from build123d import *

# Parameters (mm, degrees)
SKETCH2_R           = 3.0099
BOSS_EXTRUDE1_DEPTH = 6.0198
SKETCH3_R           = 4.5466
SKETCH3_W           = 6.223
SKETCH3_H           = 8.4836
BOSS_EXTRUDE2_DEPTH = 0.9398
SKETCH4_R           = 4.5466
BOSS_EXTRUDE3_DEPTH = 17.6022
SKETCH5_W           = 6.223
SKETCH5_H           = 8.4836
CUT_EXTRUDE1_DEPTH  = 1.8542
SKETCH6_R           = 5.969
BOSS_EXTRUDE4_DEPTH = 1.8542
SKETCH9_R           = 6.985
BOSS_EXTRUDE6_DEPTH = 2.5654
DRAFT2_ANGLE        = -25
DRAFT3_ANGLE        = -25
SKETCH12_R          = 3.8989
BOSS_EXTRUDE7_DEPTH = 25.654


with BuildPart() as part:
    # Sketch2 → Boss-Extrude1 (new body)
    with BuildSketch(Plane(origin=(0, 0, 0), x_dir=(0, 0, -1), z_dir=(1, 0, 0))):
        with BuildLine():
            ThreePointArc((-32.512356648, -30.822448246), (-32.069394739, -31.178374506), (-31.515555535, -31.3055))
            Line((-31.515555535, -31.3055), (-29.21, -31.3055))
            ThreePointArc((-29.21, -31.3055), (-28.311974388, -30.933525612), (-27.94, -30.0355))
            Line((-27.94, -30.0355), (-27.94, -23.3045))
            ThreePointArc((-27.94, -23.3045), (-24.700446352, -20.987224463), (-22.998148855, -17.3863))
            Line((-22.998148855, -17.3863), (-22.998148855, -11.1633))
            Line((-22.998148855, -11.1633), (-24.8285, -11.1633))
            Line((-24.8285, -11.1633), (-24.8285, -4.3815))
            Line((-24.8285, -4.3815), (-21.082, -4.3815))
            Line((-21.082, -4.3815), (-21.082, 11.6205))
            Line((-21.082, 11.6205), (-10.8966, 19.2405))
            Line((-10.8966, 19.2405), (10.8966, 19.2405))
            Line((10.8966, 19.2405), (21.082, 11.6205))
            Line((21.082, 11.6205), (21.082, -4.3815))
            Line((21.082, -4.3815), (24.8285, -4.3815))
            Line((24.8285, -4.3815), (24.8285, -11.1633))
            Line((24.8285, -11.1633), (22.998148855, -11.1633))
            Line((22.998148855, -11.1633), (22.998148855, -17.3863))
            ThreePointArc((22.998148855, -17.3863), (24.700446352, -20.987224463), (27.94, -23.3045))
            Line((27.94, -23.3045), (27.94, -30.0355))
            ThreePointArc((27.94, -30.0355), (28.311974388, -30.933525612), (29.21, -31.3055))
            Line((29.21, -31.3055), (31.515555535, -31.3055))
            ThreePointArc((31.515555535, -31.3055), (32.069394739, -31.178374506), (32.512356648, -30.822448246))
            Line((32.512356648, -30.822448246), (42.536992541, -18.124576114))
            ThreePointArc((42.536992541, -18.124576114), (43.315187388, -16.736717659), (43.625872471, -15.176200729))
            Line((43.625872471, -15.176200729), (44.800437362, 14.721814671))
            ThreePointArc((44.800437362, 14.721814671), (43.830873172, 17.911699115), (41.092535101, 19.813519845))
            Line((41.092535101, 19.813519845), (6.15681953, 29.583677589))
            ThreePointArc((6.15681953, 29.583677589), (0, 30.428383513), (-6.15681953, 29.583677589))
            Line((-6.15681953, 29.583677589), (-41.092535101, 19.813519845))
            ThreePointArc((-41.092535101, 19.813519845), (-43.830873172, 17.911699115), (-44.800437362, 14.721814671))
            Line((-44.800437362, 14.721814671), (-43.625872471, -15.176200729))
            ThreePointArc((-43.625872471, -15.176200729), (-43.315187388, -16.736717659), (-42.536992541, -18.124576114))
            Line((-42.536992541, -18.124576114), (-32.512356648, -30.822448246))
        make_face()
        with Locations((-34.798, 10.8585)):
            Circle(SKETCH2_R, mode=Mode.SUBTRACT)
        with Locations((34.798, 10.8585)):
            Circle(SKETCH2_R, mode=Mode.SUBTRACT)
    extrude(amount=BOSS_EXTRUDE1_DEPTH)

    # Sketch3 → Boss-Extrude2 (add)
    with BuildSketch(Plane(origin=(6.0198, 0, 0), x_dir=(0, 0, -1), z_dir=(1, 0, 0))):
        with Locations((33.9979, -16.616175495)):
            Circle(SKETCH3_R)
        with Locations((-33.9979, -16.616175495)):
            Circle(SKETCH3_R)
        with Locations((24.1935, 2.6543)):
            Rectangle(SKETCH3_W, SKETCH3_H)
        with Locations((-24.1935, 2.6543)):
            Rectangle(SKETCH3_W, SKETCH3_H)
    extrude(amount=BOSS_EXTRUDE2_DEPTH)

    # Sketch4 → Boss-Extrude3 (add)
    with BuildSketch(Plane(origin=(6.9596, 0, 0), x_dir=(0, 0, -1), z_dir=(1, 0, 0))):
        with Locations((-33.9979, -16.616175495)):
            Circle(SKETCH4_R)
        with Locations((33.9979, -16.616175495)):
            Circle(SKETCH4_R)
    extrude(amount=BOSS_EXTRUDE3_DEPTH)

    # Sketch5 → Cut-Extrude1 (cut)
    with BuildSketch(Plane.ZY):
        with Locations((-24.1935, 2.6543)):
            Rectangle(SKETCH5_W, SKETCH5_H)
        with Locations((24.1935, 2.6543)):
            Rectangle(SKETCH5_W, SKETCH5_H)
    extrude(amount=-CUT_EXTRUDE1_DEPTH, mode=Mode.SUBTRACT)

    # Sketch6 → Boss-Extrude4 (add)
    with BuildSketch(Plane.ZY):
        with Locations(Location((33.9979, -16.616175495, 0), (0, 0, 180))):
            Circle(SKETCH6_R)
        with Locations(Location((-33.9979, -16.616175495, 0), (0, 0, 180))):
            Circle(SKETCH6_R)
    extrude(amount=BOSS_EXTRUDE4_DEPTH)

    # Sketch9 → Boss-Extrude6 (add)
    with BuildSketch(Plane.ZY.offset(1.8542)):
        with Locations((33.9979, -16.616175495)):
            Circle(SKETCH9_R)
        with Locations(Location((-33.9979, -16.616175495, 0), (0, 0, 180))):
            Circle(SKETCH9_R)
    extrude(amount=BOSS_EXTRUDE6_DEPTH)

    # Draft2
    draft2_faces = [part.faces().sort_by_distance(p)[0] for p in [
        (-3.1369, -16.616175495, -27.0129),
    ]]
    draft(draft2_faces, Plane(origin=(-1.8542, -16.616175495, -33.9979), x_dir=(0, 0, 1), z_dir=(1, 0, 0)), DRAFT2_ANGLE)

    # Draft3
    draft3_faces = [part.faces().sort_by_distance(p)[0] for p in [
        (-3.1369, -16.616175495, 27.0129),
    ]]
    draft(draft3_faces, Plane(origin=(-1.8542, -16.616175495, 33.9979), x_dir=(0, 0, 1), z_dir=(1, 0, 0)), DRAFT3_ANGLE)

    # Sketch12 → Boss-Extrude7 (add)
    with BuildSketch(Plane.ZY.offset(4.4196)):
        with Locations((-33.9979, -16.616175495)):
            Circle(SKETCH12_R)
        with Locations(Location((33.9979, -16.616175495, 0), (0, 0, 180))):
            Circle(SKETCH12_R)
    extrude(amount=BOSS_EXTRUDE7_DEPTH)


solid = part.part
Read the model definition and answer for the solid it produces. Units are mm, in the model's axes. A direction names the side the tool comes from. Round coordinates to 2 decimals unless told otherwise and drop trailing zeros. Loops run counter-clockwise (first coordinate to the right, second up) from the corner with the lowest first, then second, coordinate; pieces in that order, holes last.
Q1. Each of these flat-tipped pins is pushed along its axis until it touches: pin 1 (0.8 mm diameter, centred on x = 6.5, z = -23.5, fed in from +Y); pin 2 (5 mm diameter, centred on x = 16, z = 33, fed in from -Y); pin 3 (4 mm diameter, centred on x = 1.5, z = -31.5, fed in from +Y); pin 4 (8 mm diameter, centred on x = -10.5, y = -7.5, fed in from +Z). Where does it stop, or does it pass through?
Q2. Consider probe 1 along Z at (x, y) = (5, -15.5); probe 2 along X at (y, z) = (-26, 31); probe 3 along Y at (x, z) = (17, -34). Determine where each line is inside the solid, lowest interval first.
Q3. Section A-A on y = 16.5 is taken. Write down the section's boundary in (x, z).
Q4. Section D-D on y = 25 is taken. Write down the section's boundary in (x, z), and give its area (3 significant figures).
Q5. Section C-C on y = 5.5 is taken. Write down the section's boundary in (x, z) (3 decimals).
Q6. Determine the mould class of faces 5 (the face through (2.968, -16.758, -43.307)), 6 (the face through (15.16, -13.54, -30.65)), 7 (the face through (1, 6.896, 24)) for opening direction Y: released by +Y, released by -Y, zero draft, split by the parting line, or undercut.
Q7. Section B-B on x = -10 is taken. Write down the section's boundary in (y, z), and give its area (3 significant figures).
Q8. Which of the six approach directions +Z, -Z, +X, -X, +Y, -Y give full straight-line access (tool end or side, diameter ignored) to faces 1 (the face through (-1.854, -13, 39)), 2 (the face through (2.968, -21.03, 24.737)), 3 (the face through (3, -11.163, -24)), 4 (the face through (-4.42, -18, 38))?
Output:
1. pin 1: stops at y = 6.9
1. pin 2: stops at y = -21.16
1. pin 3: stops at y = 23.06
1. pin 4: passes through
2. probe 1: z = -43.6 to -23, 23 to 43.6
2. probe 2: x = 0 to 6.02
2. probe 3: y = -21.16 to -12.07
3. outline: (0, -44.55) - (6.02, -44.55) - (6.02, -14.56) - (0, -14.56) - close; (0, 14.56) - (6.02, 14.56) - (6.02, 44.55) - (0, 44.55) - close
4. outline: (0, -22.55) - (6.02, -22.55) - (6.02, 22.55) - (0, 22.55) - close
4. area: 271 mm2
5. outline: (0, -44.438) - (6.02, -44.438) - (6.02, -27.305) - (6.96, -27.305) - (6.96, -21.082) - (1.854, -21.082) - (1.854, -27.305) - (0, -27.305) - close; (0, 27.305) - (1.854, 27.305) - (1.854, 21.082) - (6.96, 21.082) - (6.96, 27.305) - (6.02, 27.305) - (6.02, 44.438) - (0, 44.438) - close
6. face 5: released by -Y
6. face 6: split by the parting line
6. face 7: undercut
7. outline: circle Ø7.8 at (-16.62, -34); circle Ø7.8 at (-16.62, 34)
7. area: 95.5 mm2
8. face 1: none
8. face 2: +X, -X, -Y
8. face 3: +X, -X
8. face 4: -X
